Source: CAD feature listing. Evaluate the final solid. Frame: model axes, mm. Give positions to 0.01 mm unless a question says otherwise; leave off trailing zeros. Loops run counter-clockwise (first coordinate to the right, second up) from the corner with the lowest first, then second, coordinate; pieces in that order, holes last. Notation, with made-up numbers: (25, 20.5) - (56, 20.5) arc R28 ccw to (56, 59.5) - close; hole circle Ø5 at (-33, -18.75). An arc over 180 degrees is marked (long way). Put each result on its own line as item: value.
```python
from build123d import *

# Parameters (mm, degrees)
SKETCH1_R           = 112
SKETCH1_R_2         = 110
BOSS_EXTRUDE1_DEPTH = 10
SKETCH2_W           = 24
SKETCH2_H           = 6
CUT_EXTRUDE1_DEPTH  = 113
CIRPATTERN1_COUNT   = 24


with BuildPart() as part:
    # Sketch1 → Boss-Extrude1 (new body)
    with BuildSketch(Plane(origin=(0, 0, 0), x_dir=(1, 0, 0), z_dir=(0, 1, 0))):
        Circle(SKETCH1_R)
        Circle(SKETCH1_R_2, mode=Mode.SUBTRACT)
    extrude(amount=BOSS_EXTRUDE1_DEPTH)

    # Sketch2 → Cut-Extrude1 (cut, through all)
    with BuildSketch(Plane.XY):
        with Locations((-4.41590823, 5)):
            Rectangle(SKETCH2_W, SKETCH2_H)
    cut_extrude1 = extrude(amount=-CUT_EXTRUDE1_DEPTH, mode=Mode.SUBTRACT)

    # CirPattern1: Cut-Extrude1 ×24 about axis
    cirpattern1_axis = Axis((0, 0, 0), (0, 1, 0))
    for i in range(1, CIRPATTERN1_COUNT):
        add(cut_extrude1.rotate(cirpattern1_axis, i * 360 / CIRPATTERN1_COUNT), mode=Mode.SUBTRACT)


solid = part.part
```
1) Section query A-A, the plane x = 0. Output: boundary loops of the cut face in (y, z).
Check result:
outline: (0, -112) - (2, -112) - (2, -110) - (0, -110) - close; (0, 110) - (2, 110) - (2, 112) - (0, 112) - close; (8, -112) - (10, -112) - (10, -110) - (8, -110) - close; (8, 110) - (10, 110) - (10, 112) - (8, 112) - close
2) Pin query (flat end, axial travel): P1, Ø2, axis at y = 3.5, z = -109.5, coming from the +X side; P2, Ø5, axis at y = 1.5, z = -44.5, coming from the +X side; P3, Ø2, axis at x = -110, y = 4.5, coming from the -Z side. Return the tip coordinate at first contact, or that it passes through.
Check result:
P1: x = 12.61
P2: x = 103.83
P3: z = -12.75
3) Mould query, pull axis Y, two halves, no side actions, for faces 1 (the flat face through (74, 0, 82)), 2 (the flat face through (-98, 8, -51)). Classes: pulls with the +Y half, pulls with the -Y half, needs draft (parallel to the pull), parting line crosses it, or undercut.
Check result:
face 1: pulls with the -Y half
face 2: undercut
4) Section query C-C, the plane y = 4.5. State how many separate pieces and enclosed holes the cut face has, plus the area to 3 significant figures.
Check result:
separate pieces: 24
enclosed holes: 0
area: 240 mm²
5) Section query B-B, the plane z = 0. Output: boundary loops of the cut face in (x, y).
Check result:
outline: (-112, 0) - (-110, 0) - (-110, 2) - (-112, 2) - close; (-112, 8) - (-110, 8) - (-110, 10) - (-112, 10) - close; (110, 0) - (112, 0) - (112, 2) - (110, 2) - close; (110, 8) - (112, 8) - (112, 10) - (110, 10) - close
6) Material intervals for line 1 along Z through (x, y) = (94.5, 8.75); line 2 along X through (y, z) = (1.25, -95); line 3 along Z through (x, y) = (-25.5, 1.25), sorted ascending. Write a range as [from, to].
Check result:
line 1: [-60.11, -56.3], [56.3, 60.11]
line 2: [-59.32, -55.45], [55.45, 59.32]
line 3: [-109.06, -107], [107, 109.06]
